Design review of the part shown in the three views and the two pictorial views. Dimensions are in mm from the part's minimum x, y and z. Give positions to 0.01 mm unless a question says otherwise; leave off trailing zeros. Write each loop counter-clockwise with the first axis right and the second up, starting at its lowest first coordinate (ties: lowest second). Pieces come first, ordered by that corner, then holes.
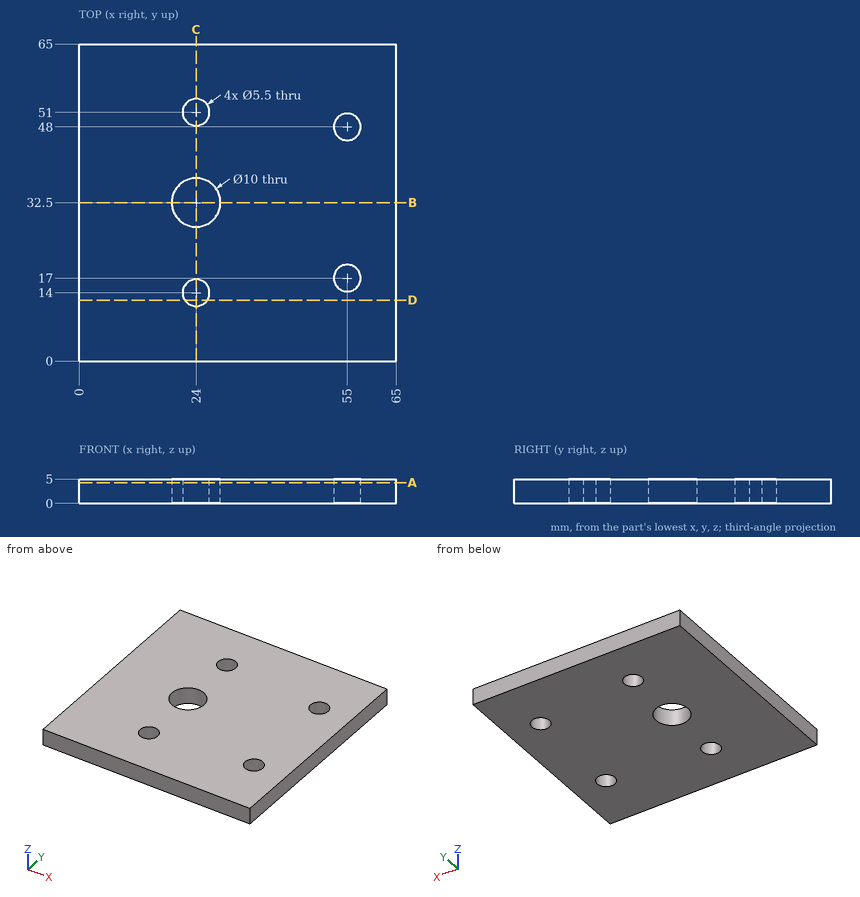
(1) Clearance check with flat-ended pins moving along their axes: P1, Ø4.5, axis at x = 24, y = 14, coming from the -Z side; P2, Ø2, axis at y = 27.5, z = 3.5, coming from the -X side. State where each tip first meets the part, or that it passes through.
Resolved:
P1: passes through
P2: stops at x = 0
(2) Consider section B-B, the plane y = 32.5. Give the boundary of the cut face in (x, z).
Resolved:
outline: (0, 0) - (19, 0) - (19, 5) - (0, 5) - close; (29, 0) - (65, 0) - (65, 5) - (29, 5) - close
(3) To check wall thickness, follow L1, parallel to Y at x = 24, z = 2.4; L2, parallel to Y at x = 55, z = 2.2; L3, parallel to Y at x = 22.5, z = 1.8. State the ranges of each line that lie inside material, in increasing order.
Resolved:
L1: y = 0 to 11.25, 16.75 to 27.5, 37.5 to 48.25, 53.75 to 65
L2: y = 0 to 14.25, 19.75 to 45.25, 50.75 to 65
L3: y = 0 to 11.7, 16.3 to 27.73, 37.27 to 48.7, 53.3 to 65
(4) Consider section D-D, the plane y = 12.5. Give the boundary of the cut face in (x, z), then the cut area to 3 significant figures.
Resolved:
outline: (0, 0) - (21.7, 0) - (21.7, 5) - (0, 5) - close; (26.3, 0) - (65, 0) - (65, 5) - (26.3, 5) - close
area: 302 mm2
(5) Consider section C-C, the plane x = 24. Give the boundary of the cut face in (y, z), then the cut area to 3 significant figures.
Resolved:
outline: (0, 0) - (11.25, 0) - (11.25, 5) - (0, 5) - close; (16.75, 0) - (27.5, 0) - (27.5, 5) - (16.75, 5) - close; (37.5, 0) - (48.25, 0) - (48.25, 5) - (37.5, 5) - close; (53.75, 0) - (65, 0) - (65, 5) - (53.75, 5) - close
area: 220 mm2
(6) Consider section A-A, the plane z = 4.25. Give the boundary of the cut face in (x, y).
Resolved:
outline: (0, 0) - (65, 0) - (65, 65) - (0, 65) - close; hole circle Ø10 at (24, 32.5); hole circle Ø5.5 at (24, 14); hole circle Ø5.5 at (24, 51); hole circle Ø5.5 at (55, 17); hole circle Ø5.5 at (55, 48)
